```python
from build123d import *

# Parameters (mm, degrees)
F1_DEPTH = 25
F3_D     = 12
F4_SIZE2 = 24
F4_SIZE  = 9


with BuildPart() as f1:
    # F0 (on Front) → F1 (new body)
    with BuildSketch(Plane.XZ):
        Polygon((10, 30.314465), (10, 0), (0, 0), (0, -9.685535), (20, -9.685535), (20, 30.314465), align=None)
    extrude(amount=-F1_DEPTH)

    # F3 (through all)
    with Locations(Plane.YZ.offset(20)):
        with Locations((13.475935, 17.546792)):
            Hole(F3_D / 2)

    # F4
    f4_edges = [f1.edges().sort_by_distance(p)[0] for p in [
        (15, 0, 30.314465),
    ]]
    chamfer(f4_edges, length=F4_SIZE, length2=F4_SIZE2)

    # F5: F1 across plane


with BuildPart() as f1_1:
    add(f1.part)
    add(f1.part.mirror(Plane.YZ))


solid = f1_1.part
```
Source: CAD feature listing. Evaluate the final solid. Frame: model axes, mm. A direction names the side the tool comes from. Give positions to 0.01 mm unless a question says otherwise; leave off trailing zeros. Loops run counter-clockwise (first coordinate to the right, second up) from the corner with the lowest first, then second, coordinate; pieces in that order, holes last. Notation, with made-up numbers: M -33,86.25 L 8,86.25 A28 ccw 8,105.25 Z; hole C -2.5,25 d11. An arc over 180 degrees is marked long. Put each result on its own line as item: value.
Q1. Section C-C (z = 15.5). Return the cut outline in (x, y).
Response values:
outline: M -20,3.44 L -10,3.44 L -10,7.84 L -20,7.84 Z; M -20,19.12 L -10,19.12 L -10,25 L -20,25 Z; M 10,3.44 L 20,3.44 L 20,7.84 L 10,7.84 Z; M 10,19.12 L 20,19.12 L 20,25 L 10,25 Z
Q2. Section D-D (y = 14). Return the cut outline in (x, z), and give its area (3 significant figures).
Response values:
outline: M -20,-9.69 L 20,-9.69 L 20,11.57 L 10,11.57 L 10,0 L -10,0 L -10,11.57 L -20,11.57 Z; M -20,23.52 L -10,23.52 L -10,30.31 L -20,30.31 Z; M 10,23.52 L 20,23.52 L 20,30.31 L 10,30.31 Z
area: 755 mm²
Q3. Section A-A (z = 5). Return the cut outline in (x, y), and give its area (3 significant figures).
Response values:
outline: M -20,0 L -10,0 L -10,25 L -20,25 Z; M 10,0 L 20,0 L 20,25 L 10,25 Z
area: 500 mm²
Q4. Section B-B (y = 20.25). Return the cut outline in (x, z).
Response values:
outline: M -20,-9.69 L 20,-9.69 L 20,30.31 L 10,30.31 L 10,0 L -10,0 L -10,30.31 L -20,30.31 Z
Q5. Pin query (flat end, axial travel): P1, Ø5, axis at x = 10.5, z = 10.5, coming from the -Y side; P2, Ø4, axis at x = -14, z = 23, coming from the -Y side. Return the tip coordinate at first contact, or that it passes through.
Response values:
P1: stops at y = 0.63
P2: stops at y = 5.51
Q6. Reachability of faces 4 (the flat face through (0, 12, 0)), 5 (the cylindrical face through (14.93, 18.24, 13.9)) from +Z, -Z, +X, -X, +Y, -Y: full face, straight path, thin tool, end or side. Return the list, or none.
Response values:
face 4: +Z, +Y, -Y
face 5: +X, -X
Q7. Line query: probe 1 along X at (y, z) = (9.25, 25.5); probe 2 along Z at (x, y) = (-5, 14.5); probe 3 along Z at (x, y) = (17, 18.5). Output: solid intervals per line, ascending. Write a range as [from, to].
Response values:
probe 1: x = [-20, -10], [10, 20]
probe 2: z = [-9.69, 0]
probe 3: z = [-9.69, 14.27], [20.83, 30.31]
Q8. Mould query, pull axis X, two halves, no side actions, for faces 1 (the flat face through (-15.07, 4.44, 18.15)), 2 (the flat face through (-10, 18, 12)), 3 (the flat face through (-20, 12, 6)). Classes: released by +X, released by -X, zero draft, split by the parting line, or undercut.
Response values:
face 1: zero draft
face 2: undercut
face 3: released by -X
